Build history of the part. All positions in model axes, mm. Round coordinates to 2 decimals unless told otherwise and drop trailing zeros. Order: outer loops, then holes, each group sorted by start corner. A loop starts at its lowest first (then second) coordinate and runs counter-clockwise, first axis right, second up. Notation, with made-up numbers: M 0,78 L 29,78 A21 ccw 29,101 Z; hole C 79,52 d10. An arc over 180 degrees is marked long. Use CSV: the item, a comma, the result in double quotes.
from build123d import *

# Parameters (mm, degrees)
SKETCH1_W           = 120
SKETCH1_H           = 15
SKETCH1_R           = 5
SKETCH1_R_2         = 1.5
BOSS_EXTRUDE1_DEPTH = 2
FILLET1_R           = 1


with BuildPart() as part:
    # Sketch1 → Boss-Extrude1 (new body)
    with BuildSketch(Plane(origin=(0, 0, 0), x_dir=(1, 0, 0), z_dir=(0, 1, 0))):
        with Locations((60, 7.5)):
            Rectangle(SKETCH1_W, SKETCH1_H)
        with Locations(Location((10, 7.5, 0), (0, 0, 270))):
            Circle(SKETCH1_R, mode=Mode.SUBTRACT)
        with Locations(Location((110, 7.5, 0), (0, 0, 270))):
            Circle(SKETCH1_R, mode=Mode.SUBTRACT)
        with Locations(Location((50, 7.5, 0), (0, 0, 270))):
            Circle(SKETCH1_R_2, mode=Mode.SUBTRACT)
        with Locations(Location((70, 7.5, 0), (0, 0, 270))):
            Circle(SKETCH1_R_2, mode=Mode.SUBTRACT)
    extrude(amount=BOSS_EXTRUDE1_DEPTH)

    # Fillet1
    fillet1_edges = [part.edges().sort_by_distance(p)[0] for p in [
        (120, 1, 0),
        (0, 1, 0),
        (0, 1, -15),
        (120, 1, -15),
    ]]
    fillet(fillet1_edges, radius=FILLET1_R)


solid = part.part
(1) Cut at D-D, the plane x = 110. Give the cut face in (y, z).
Answer block:
outline,"M 0,-15 L 2,-15 L 2,-12.5 L 0,-12.5 Z; M 0,-2.5 L 2,-2.5 L 2,0 L 0,0 Z"
(2) Drop a flat-ended pin along its axis: pin 1 (1.8 mm diameter, centred on x = 70, z = -7.5, fed in from -Y). Give the stop position or say it passes through.
Answer block:
pin 1,"passes through"
(3) Cut at B-B, the plane y = 0.6. Give the cut face in (x, z), and give its area (3 significant figures).
Answer block:
outline,"M 0,-14 A1 ccw 1,-15 L 119,-15 A1 ccw 120,-14 L 120,-1 A1 ccw 119,0 L 1,0 A1 ccw 0,-1 Z; hole C 10,-7.5 d10; hole C 50,-7.5 d3; hole C 70,-7.5 d3; hole C 110,-7.5 d10"
area,"1,630 mm²"
(4) Two-plate mould, pull along Z, no slides. Class faces 1 (the face through (59, 0, -8)), 2 (the face through (11.5, 0.99, -2.73)), 3 (the face through (59, 1, -15)), 4 (the face through (59, 1, 0)): released by +Z, released by -Z, zero draft, split by the parting line, or undercut.
Answer block:
face 1,"zero draft"
face 2,"undercut"
face 3,"released by -Z"
face 4,"released by +Z"
(5) Cut at A-A, the plane z = -7.5. Give the cut face in (x, y).
Answer block:
outline,"M 0,0 L 5,0 L 5,2 L 0,2 Z; M 15,0 L 48.5,0 L 48.5,2 L 15,2 Z; M 51.5,0 L 68.5,0 L 68.5,2 L 51.5,2 Z; M 71.5,0 L 105,0 L 105,2 L 71.5,2 Z; M 115,0 L 120,0 L 120,2 L 115,2 Z"
(6) Wall check: line 1 (X direction, y = 0.9, z = -7.25); line 2 (X direction, y = 1.8, z = -4.25); line 3 (Z direction, x = 70, y = 0.7). Give the ranges that are in metal, low to high. Write a range as from..to.
Answer block:
line 1,"x = 0..5.01, 14.99..48.52, 51.48..68.52, 71.48..105.01, 114.99..120"
line 2,"x = 0..6.2, 13.8..106.2, 113.8..120"
line 3,"z = -15..-9, -6..0"
(7) Cut at C-C, the plane x = 50. Give the cut face in (y, z), and give its area (3 significant figures).
Answer block:
outline,"M 0,-15 L 2,-15 L 2,-9 L 0,-9 Z; M 0,-6 L 2,-6 L 2,0 L 0,0 Z"
area,"24.0 mm²"
